Verification items for the finished model (mm, model axes). A direction names the side the tool comes from. Round coordinates to 2 decimals unless told otherwise and drop trailing zeros. Write each loop counter-clockwise with the first axis right and the second up, starting at its lowest first coordinate (ties: lowest second). Pieces come first, ordered by that corner, then holes. Notation, with made-up numbers: (22, 87.5) - (53, 87.5) arc R28 ccw to (53, 120.5) - close; hole circle Ø8 at (19.25, 40). An arc over 180 degrees is marked (long way). Answer as a JSON object with one key per item and string values. Group by question number.
1) Section check D-D (x = -43). State how many separate pieces and enclosed holes the cut face has, then the cut area to 3 significant figures.
2) Section check C-C (z = 35). Enter the section's corners in (x, y), then the cut area to 3 significant figures.
3) Thickness scan on line 1 (Y direction, x = 31.5, z = 56); line 2 (X direction, y = -14, z = 77.5); line 3 (X direction, y = -12, z = 26.5) (3 decimals). Record the ranges inside material, lowest first.
4) Mould release check, pull along Y, two halves, no side actions. Record for faces 1 (the cylindrical face through (-101.61, 51.3, 13.33)), 2 (the flat face through (-94, -29, 25.4)), 3 (the conical face through (45.542, 71.432, 45.01)): +Y half, -Y half, draft (parallel to the pull), parting line (faces both ways), or undercut.
5) Go/stop test with flat-tipped pins: pin 1 Ø5 at (y, z) = (-44, 46.5) entering from -X; pin 2 Ø10 at (x, z) = (27, 78.5) entering from +Y; pin 3 Ø12 at (x, z) = (68.5, 57) entering from +Y. Record where each tip stops, or that it passes through.
6) Set-up check for faces 4 (the cylindrical face through (-18.239, -82.137, 65.607)), 5 (the flat face through (-60.7, -91.4, 1.588)), 6 (the cylindrical face through (101.61, -51.3, 13.33)): record each of +Z, -Z, +X, -X, +Y, -Y from which the full face is reachable in a straight line by a thin tool's end or side.
```python
from build123d import *

# Parameters (mm, degrees)
SKETCH1_R                 = 139.7
BOSS_EXTRUDE1_DEPTH       = 25.4
SKETCH2_R                 = 11.1125
BOLTHOLE_DEPTH            = 200.191716695
BOLTHOLEPATTERN_COUNT     = 8
SKETCH5_OUTSIDE_W         = 360.59
SKETCH5_OUTSIDE_H         = 360.59
SKETCH5_OUTSIDE_R         = 107.95
RAISED_FACE_DEPTH         = 1.5875
SKETCH8_R                 = 96.0374
WELD_NECK_120_DRAFT_DEPTH = 63.5
WELD_NECK_120_DRAFT_TAPER = 30
WELD_NECK_END_REACH       = 218.646
SKETCH9_R                 = 84.1375
WELD_NECK_CHAMFER1_SIZE   = 4.239097945
WELD_NECK_CHAMFER1_SIZE2  = 5.5245
SKETCH7_R                 = 77.0255
BORE_DEPTH                = 217.645770787
FILLET2_R                 = 1.5875
FILLET3_R                 = 1.5875


with BuildPart() as part:
    # Sketch1 → Boss-Extrude1 (new body)
    with BuildSketch(Plane.XY):
        Circle(SKETCH1_R)
    extrude(amount=BOSS_EXTRUDE1_DEPTH)

    # Sketch2 → BoltHole (cut, through all)
    with BuildSketch(Plane.XY):
        with Locations((46.170756115, 111.466065597)):
            Circle(SKETCH2_R)
    bolthole = extrude(amount=BOLTHOLE_DEPTH, mode=Mode.SUBTRACT)

    # BoltHolePattern: BoltHole ×8 about axis
    boltholepattern_axis = Axis((0, 0, 0), (0, 0, 1))
    for i in range(1, BOLTHOLEPATTERN_COUNT):
        add(bolthole.rotate(boltholepattern_axis, i * 360 / BOLTHOLEPATTERN_COUNT), mode=Mode.SUBTRACT)

    # Sketch5 outside → Raised Face (cut)
    with BuildSketch(Plane(origin=(0, 0, 0), x_dir=(-1, 0, 0), z_dir=(0, 0, -1))):
        Rectangle(SKETCH5_OUTSIDE_W, SKETCH5_OUTSIDE_H)
        Circle(SKETCH5_OUTSIDE_R, mode=Mode.SUBTRACT)
    extrude(amount=-RAISED_FACE_DEPTH, mode=Mode.SUBTRACT)

    # Sketch8 → Weld Neck 120 Draft (add)
    with BuildSketch(Plane.XY.offset(25.4)):
        Circle(SKETCH8_R)
    extrude(amount=WELD_NECK_120_DRAFT_DEPTH, taper=WELD_NECK_120_DRAFT_TAPER)

    # Sketch9 → Weld Neck End (add, up to next)
    with BuildSketch(Plane.XY.offset(88.9), mode=Mode.PRIVATE) as weld_neck_end_sk1:
        Circle(SKETCH9_R)
    weld_neck_end_tool1 = extrude(weld_neck_end_sk1.sketch, amount=-WELD_NECK_END_REACH, mode=Mode.PRIVATE) - part.part
    add(weld_neck_end_tool1.solids().sort_by_distance((0, 0, 88.9))[0])

    # Weld Neck Chamfer1
    weld_neck_chamfer1_edges = [part.edges().sort_by_distance(p)[0] for p in [
        (-84.1375, 0, 88.9),
    ]]
    weld_neck_chamfer1_side = [part.faces().sort_by_distance(p)[0] for p in [
        (-84.1375, 0, 67.455615702),
    ]]
    chamfer(weld_neck_chamfer1_edges, length=WELD_NECK_CHAMFER1_SIZE, length2=WELD_NECK_CHAMFER1_SIZE2, reference=weld_neck_chamfer1_side[0])

    # Sketch7 → Bore (cut, through all)
    with BuildSketch(Plane.XY):
        Circle(SKETCH7_R)
    extrude(amount=BORE_DEPTH, mode=Mode.SUBTRACT)

    # Fillet2
    fillet2_edges = [part.edges().sort_by_distance(p)[0] for p in [
        (-139.7, 0, 25.4),
        (-139.7, 0, 1.5875),
    ]]
    fillet(fillet2_edges, radius=FILLET2_R)

    # Fillet3
    fillet3_edges = [part.edges().sort_by_distance(p)[0] for p in [
        (107.95, 0, 1.5875),
    ]]
    fillet(fillet3_edges, radius=FILLET3_R - 0.0001)  # a hair under: the kernel refuses the full size


solid = part.part
```
Returned:
{
 "1": {"separate pieces": "4", "enclosed holes": "0", "area": "3,700 mm2"},
 "2": {"outline": "circle Ø180.99 at (0, 0); hole circle Ø154.05 at (0, 0)", "area": "7,090 mm2"},
 "3": {"line 1": "-78.02 to -70.29, 70.29 to 78.02", "line 2": "-82.96 to -75.74, 75.74 to 82.96", "line 3": "-94.645 to -76.085, 76.085 to 94.645"},
 "4": {"face 1": "undercut", "face 2": "draft", "face 3": "parting line"},
 "5": {"pin 1": "x = -73.63", "pin 2": "y = 81.21", "pin 3": "y = 56.33"},
 "6": {"face 4": "+Z", "face 5": "-Z", "face 6": "+Z, -Z"}
}
